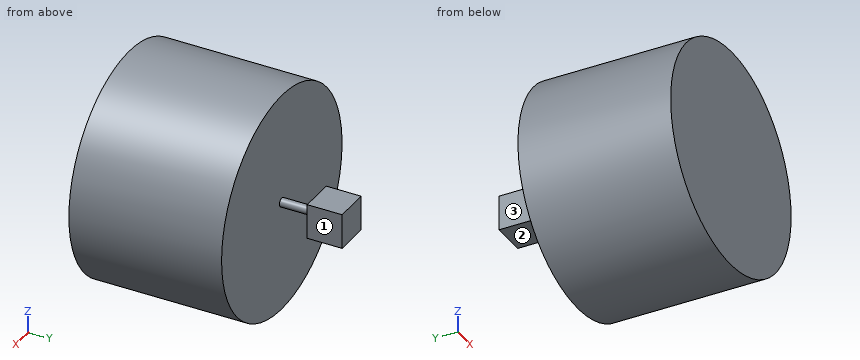
```python
from build123d import *

# Parameters (mm, degrees)
ESQUISSE1_R      = 254
EXTRUSION1_DEPTH = 350
ESQUISSE2_R      = 10
EXTRUSION2_DEPTH = 80
ESQUISSE3_W      = 80
ESQUISSE3_H      = 80
EXTRUSION3_DEPTH = 80


with BuildPart() as part:
    # Esquisse1 → Extrusion1 (new body)
    with BuildSketch(Plane(origin=(0, 0, 0), x_dir=(1, 0, 0), z_dir=(0, 1, 0))):
        Circle(ESQUISSE1_R)
    extrude(amount=EXTRUSION1_DEPTH)

    # Esquisse2 → Extrusion2 (add)
    with BuildSketch(Plane(origin=(0, 350, 0), x_dir=(1, 0, 0), z_dir=(0, 1, 0))):
        Circle(ESQUISSE2_R)
    extrude(amount=EXTRUSION2_DEPTH)

    # Esquisse3 → Extrusion3 (add)
    with BuildSketch(Plane(origin=(0, 430, 0), x_dir=(1, 0, 0), z_dir=(0, 1, 0))):
        Rectangle(ESQUISSE3_W, ESQUISSE3_H)
    extrude(amount=EXTRUSION3_DEPTH)


solid = part.part
```
Here's how the part is built. I have some questions about the finished solid (model axes, mm). Face numbers are marked on the shaded views. A direction names the side the tool comes from. Coordinates: 2 decimals unless noted, no trailing zeros. Loops run counter-clockwise (first coordinate to the right, second up) from the corner with the lowest first, then second, coordinate; pieces in that order, holes last. Notation, with made-up numbers: (37.25, 85) - (45.25, 85) arc R18 ccw to (45.25, 120) - close; hole circle Ø9 at (45, 68). An arc over 180 degrees is marked (long way). Answer as CSV lines item,"result".
Q1. For pin 1 (10 mm diameter, centred on x = -187, y = 139, fed in from -Z); pin 2 (12 mm diameter, centred on x = -40.5, z = -202, fed in from +Y); pin 3 (12 mm diameter, centred on y = 284.5, z = 133.5, fed in from -X), each with a flat end and sliding along its axis, tell me the tip position at first contact or that it passes through.
Response:
pin 1,"z = -177.18"
pin 2,"y = 350"
pin 3,"x = -219.68"
Q2. If I drill on L1, parallel to Y at x = 30, z = 22; L2, parallel to Y at x = 10.5, z = -177; L3, parallel to Z at x = 38, y = 483, over which ranges is the centre line in solid material (lowest first)? Write a range as [from, to].
Response:
L1,"[0, 350], [430, 510]"
L2,"[0, 350]"
L3,"[-40, 40]"
Q3. For the marked faces 1, 2 and 3, which set-ups out of +Z, -Z, +X, -X, +Y, -Y let a thin tool reach every point of the face, with its end or its side?
Response:
face 1,"+Z, -Z, +X, +Y"
face 2,"-Z, +X, -X, +Y"
face 3,"+Z, -Z, -X, +Y"
Q4. If we section it at A-A, the plane x = 0: Write out the boundary of the cut face in (y, z).
Response:
outline,"(0, -254) - (350, -254) - (350, -10) - (430, -10) - (430, -40) - (510, -40) - (510, 40) - (430, 40) - (430, 10) - (350, 10) - (350, 254) - (0, 254) - close"
Q5. If we section it at D-D, the plane y = 408: Write out the boundary of the cut face in (x, z).
Response:
outline,"circle Ø20 at (0, 0)"
Q6. If we section it at B-B, the plane z = 0: Write out the boundary of the cut face in (x, y), and give its area (3 significant figures).
Response:
outline,"(-254, 0) - (254, 0) - (254, 350) - (10, 350) - (10, 430) - (40, 430) - (40, 510) - (-40, 510) - (-40, 430) - (-10, 430) - (-10, 350) - (-254, 350) - close"
area,"186,000 mm2"
Q7. If we section it at C-C, the plane y = 116: Write out the boundary of the cut face in (x, z).
Response:
outline,"circle Ø508 at (0, 0)"
